Verification items for the finished model (mm, model axes). A direction names the side the tool comes from. Coordinates: 2 decimals unless noted, no trailing zeros. Write each loop counter-clockwise with the first axis right and the second up, starting at its lowest first coordinate (ties: lowest second). Pieces come first, ordered by that corner, then holes. Notation, with made-up numbers: (27.25, -28.75) -> (38.25, -28.75) arc R8 cw to (38.25, -19.75) -> close; hole circle Ø5 at (49.5, 42.5). An arc over 180 degrees is marked (long way). Answer in a Markdown table with one row per item.
```python
from build123d import *

# Parameters (mm, degrees)
SKETCH1_W             = 19
SKETCH1_H             = 7.4
BOSS_EXTRUDE1_DEPTH   = 18
SKETCH1_H_2           = 5.8
BOSS_EXTRUDE1_2_DEPTH = 18
SKETCH1_6_W           = 12.45
SKETCH1_6_H           = 5.8
BOSS_EXTRUDE6_DEPTH   = 38
BOSS_EXTRUDE7_DEPTH   = 10
SKETCH4_W             = 18
SKETCH4_H             = 7.4
SKETCH4_H_2           = 5.8
BOSS_EXTRUDE8_DEPTH   = 3
CUT_EXTRUDE1_START    = -7.4
SKETCH6_R             = 1.5
CUT_EXTRUDE1_DEPTH    = 20
BOSS_EXTRUDE10_REACH  = 46.586
SKETCH7_W             = 2
SKETCH7_H             = 38
BOSS_EXTRUDE11_REACH  = 47.064
SKETCH8_W             = 7.5
SKETCH8_H             = 3
SKETCH9_R             = 2
CUT_EXTRUDE2_DEPTH    = 2
CUT_EXTRUDE3_START    = -10.45
CUT_EXTRUDE3_DEPTH    = 8.45


# Read off the part's stored shape, not the designer's step: Cut-Extrude3
with BuildPart() as part:
    # Sketch1 → Boss-Extrude1 (new body)
    with BuildSketch(Plane.XY):
        with Locations((7.125, 0)):
            Rectangle(SKETCH1_W, SKETCH1_H)
    extrude(amount=-BOSS_EXTRUDE1_DEPTH)



with BuildPart() as body_2:
    # Sketch1 → Boss-Extrude1 2 (new body)
    with BuildSketch(Plane.XY):
        with Locations((7.125, 13.4)):
            Rectangle(SKETCH1_W, SKETCH1_H_2)
    extrude(amount=-BOSS_EXTRUDE1_2_DEPTH)


with BuildPart() as part_1:
    add(part.part)

    add(body_2.part)  # Boss-Extrude6 merges body 2
    # Sketch1<6> → Boss-Extrude6 (add)
    with BuildSketch(Plane.XY):
        Polygon((-14.825, 3.7), (-14.825, -0.7), (-9.825, -0.7), (-9.825, -3.7), (-2.375, -3.7), (-2.375, 3.7), align=None)
        with Locations((-8.6, 13.4)):
            Rectangle(SKETCH1_6_W, SKETCH1_6_H)
    extrude(amount=-BOSS_EXTRUDE6_DEPTH)

    # Sketch1<7> → Boss-Extrude7 (add)
    with BuildSketch(Plane.XY):
        Polygon((-14.825, -0.7), (-14.825, -2), (-14.825, -3.7), (-9.825, -3.7), (-9.825, -0.7), align=None)
    extrude(amount=-BOSS_EXTRUDE7_DEPTH)

    # Sketch4 → Boss-Extrude8 (add)
    with BuildSketch(Plane(origin=(16.625, 0, 0), x_dir=(0, 0, -1), z_dir=(1, 0, 0))):
        with Locations((9, 0)):
            Rectangle(SKETCH4_W, SKETCH4_H)
        with Locations((9, 13.4)):
            Rectangle(SKETCH4_W, SKETCH4_H_2)
    extrude(amount=BOSS_EXTRUDE8_DEPTH)

    # Sketch6 → Cut-Extrude1 (cut)
    with BuildSketch(Plane(origin=(0, 3.7, 0), x_dir=(1, 0, 0), z_dir=(0, 1, 0)).offset(CUT_EXTRUDE1_START)):
        with Locations(Location((10.44201924, 11.5, 0), (0, 0, 270))):
            Circle(SKETCH6_R)
    extrude(amount=CUT_EXTRUDE1_DEPTH, mode=Mode.SUBTRACT)

    # Sketch7 → Boss-Extrude10 (add, up to next)
    with BuildSketch(Plane(origin=(0, 3.7, 0), x_dir=(1, 0, 0), z_dir=(0, 1, 0)), mode=Mode.PRIVATE) as boss_extrude10_sk1:
        with Locations((-3.375, 19)):
            Rectangle(SKETCH7_W, SKETCH7_H)
    boss_extrude10_tool1 = extrude(boss_extrude10_sk1.sketch, amount=BOSS_EXTRUDE10_REACH, mode=Mode.PRIVATE) - part_1.part
    # Sketch7 → Boss-Extrude10 (add, up to next)
    with BuildSketch(Plane(origin=(0, 3.7, 0), x_dir=(1, 0, 0), z_dir=(0, 1, 0)), mode=Mode.PRIVATE) as boss_extrude10_sk2:
        with Locations((-13.825, 19)):
            Rectangle(SKETCH7_W, SKETCH7_H)
    boss_extrude10_tool2 = extrude(boss_extrude10_sk2.sketch, amount=BOSS_EXTRUDE10_REACH, mode=Mode.PRIVATE) - part_1.part
    add(boss_extrude10_tool1.solids().sort_by_distance((-3.375, 3.7, -19))[0])
    add(boss_extrude10_tool2.solids().sort_by_distance((-13.825, 3.7, -19))[0])

    # Sketch8 → Boss-Extrude11 (add, up to next)
    with BuildSketch(Plane.XZ.offset(-10.5), mode=Mode.PRIVATE) as boss_extrude11_sk1:
        with Locations((15.875, -1.5)):
            Rectangle(SKETCH8_W, SKETCH8_H)
    boss_extrude11_tool1 = extrude(boss_extrude11_sk1.sketch, amount=BOSS_EXTRUDE11_REACH, mode=Mode.PRIVATE) - part_1.part
    add(boss_extrude11_tool1.solids().sort_by_distance((15.875, 10.5, -1.5))[0])

    # Sketch9 → Cut-Extrude2 (cut)
    with BuildSketch(Plane.ZY.offset(14.825)):
        with Locations(Location((-8.095100141, 5.909535031, 0), (0, 0, 270))):
            Circle(SKETCH9_R)
    extrude(amount=-CUT_EXTRUDE2_DEPTH, mode=Mode.SUBTRACT)

    # Cut-Extrude3 outline → Cut-Extrude3 (cut)
    with BuildSketch(Plane.ZY.offset(14.825).offset(CUT_EXTRUDE3_START)):
        with BuildLine():
            Line((-4.174901811, 3.7), (-13.196516677, 3.7))
            Line((-13.196516677, 3.7), (-9.744129164, 1.722566762))
            ThreePointArc((-9.744129164, 1.722566762), (-6.589406594, 1.668911616), (-4.174901811, 3.7))
        make_face()
    extrude(amount=CUT_EXTRUDE3_DEPTH, mode=Mode.SUBTRACT)


solid = part_1.part
```
1. Section check A-A, the plane y = 9.75. Record the boundary of the cut face in (x, z) (3 decimals), plus the area to 4 significant figures.
Geometry says:
| item | result |
|---|---|
| outline | (-14.825, -38) -> (-12.825, -38) -> (-12.825, 0) -> (-14.825, 0) -> close; (-4.375, -38) -> (-2.375, -38) -> (-2.375, 0) -> (-4.375, 0) -> close; (12.125, -3) -> (19.625, -3) -> (19.625, 0) -> (12.125, 0) -> close |
| area | 174.5 mm^2 |
2. Depth check by flat-ended pin: P1, Ø3.5, axis at y = -2.5, z = -22, coming from the -X side (3 decimals); P2, Ø4.5, axis at x = 6.5, y = 14.5, coming from the -Z side; P3, Ø6, axis at y = 7, z = -15.5, coming from the +X side (3 decimals). Enter the tip coordinate at first touch or a pass-through.
Geometry says:
| item | result |
|---|---|
| P1 | x = -9.825 |
| P2 | z = -18 |
| P3 | x = -2.375 |
3. Section check B-B, the plane x = -12. Record the boundary of the cut face in (y, z).
Geometry says:
| item | result |
|---|---|
| outline | (-3.7, -10) -> (-0.7, -10) -> (-0.7, -38) -> (3.7, -38) -> (3.7, -13.2) -> (1.72, -9.74) arc R4.5 cw to (3.7, -4.17) -> (3.7, 0) -> (-3.7, 0) -> close; (10.5, -38) -> (16.3, -38) -> (16.3, 0) -> (10.5, 0) -> close |
4. Mould release check, pull along Y, two halves, no side actions. Record for faces 6 (the flat face through (-4.375, 7, -19)), 7 (the flat face through (12.125, 7, -2)), 8 (the flat face through (-9.825, -2, -24)), 9 (the flat face through (-12, -0.7, -24)): released by +Y, released by -Y, zero draft, split by the parting line, or undercut.
Geometry says:
| item | result |
|---|---|
| face 6 | undercut |
| face 7 | undercut |
| face 8 | zero draft |
| face 9 | released by -Y |
5. Section check D-D, the plane y = 5. Record the boundary of the cut face in (x, z) (3 decimals).
Geometry says:
| item | result |
|---|---|
| outline | (-14.825, -38) -> (-12.825, -38) -> (-12.825, -9.876) -> (-14.825, -9.876) -> close; (-14.825, -6.314) -> (-12.825, -6.314) -> (-12.825, 0) -> (-14.825, 0) -> close; (-4.375, -38) -> (-2.375, -38) -> (-2.375, 0) -> (-4.375, 0) -> close; (12.125, -3) -> (19.625, -3) -> (19.625, 0) -> (12.125, 0) -> close |
6. Section check C-C, the plane z = -24. Record the boundary of the cut face in (x, y) (3 decimals), plus the area to 3 significant figures.
Geometry says:
| item | result |
|---|---|
| outline | (-14.825, -0.7) -> (-9.825, -0.7) -> (-9.825, -3.7) -> (-2.375, -3.7) -> (-2.375, 16.3) -> (-14.825, 16.3) -> close; hole (-12.825, 3.7) -> (-4.375, 3.7) -> (-4.375, 10.5) -> (-12.825, 10.5) -> close |
| area | 177 mm^2 |
7. Tool access check on faces 1 (the flat face through (8, 10.5, -9)), 2 (the cylindrical face through (-13.839, 7.908, -8.007)), 3 (the flat face through (-9, 3.7, -2)), 4 (the flat face through (-8.541, 2.725, -11.494)), 5 (the flat face through (-12, -2, -10)). Record the directions out of +Z, -Z, +X, -X, +Y, -Y that give a thin tool (end or side, any length) a straight path to the whole face; none if there is none.
Geometry says:
| item | result |
|---|---|
| face 1 | -Z |
| face 2 | -X |
| face 3 | +Z, -Z |
| face 4 | none |
| face 5 | -Z, -X, -Y |
8. Thickness scan on line 1 (X direction, y = 9.5, z = -2) (3 decimals); line 2 (Y direction, x = -11, z = -17); line 3 (X direction, y = 9.25, z = -5) (3 decimals). Record the ranges inside material, lowest first. Write a range as from..to.
Geometry says:
| item | result |
|---|---|
| line 1 | -14.825..-12.825, -4.375..-2.375, 12.125..19.625 |
| line 2 | -0.7..3.7, 10.5..16.3 |
| line 3 | -14.825..-12.825, -4.375..-2.375 |
